Verification items for the finished model (mm, model axes). A direction names the side the tool comes from. Coordinates: 2 decimals unless noted, no trailing zeros. Write each loop counter-clockwise with the first axis right and the second up, starting at its lowest first coordinate (ties: lowest second). Pieces come first, ordered by that corner, then holes. Notation, with made-up numbers: (-16, 27) - (-1, 27) arc R30 ccw to (-1, 66) - close; hole circle Ø5 at (29, -1.5). An arc over 180 degrees is marked (long way). Use CSV: the item, a comma, the result in double quotes. Start each with the question number.
```python
from build123d import *

# Parameters (mm, degrees)
SKETCH1_W          = 6.5
SKETCH1_H          = 15
SKETCH2_R          = 4.5
CUT_EXTRUDE1_DEPTH = 13
SKETCH3_R          = 2
CUT_EXTRUDE2_DEPTH = 13


with BuildPart() as part:
    # Sketch1 → Revolve1 (revolve)
    with BuildSketch(Plane.XY, mode=Mode.PRIVATE) as revolve1_sk:
        with Locations((3.25, 0)):
            Rectangle(SKETCH1_W, SKETCH1_H)
    revolve(revolve1_sk.sketch.rotate(Axis((0, 7.5, 0), (0, -1, 0)), 90), axis=Axis((0, 7.5, 0), (0, -1, 0)))

    # Sketch2 → Cut-Extrude1 (cut)
    with BuildSketch(Plane.XZ.offset(7.5)):
        with Locations(Location((0, 0, 0), (0, 0, 270))):
            Circle(SKETCH2_R)
    extrude(amount=-CUT_EXTRUDE1_DEPTH, mode=Mode.SUBTRACT)

    # Sketch3 → Cut-Extrude2 (cut)
    with BuildSketch(Plane.XY):
        Circle(SKETCH3_R)
    extrude(amount=-CUT_EXTRUDE2_DEPTH, mode=Mode.SUBTRACT)


solid = part.part
```
Q1. Scan lines: line 1 along Y through (x, z) = (0, -5.1); line 2 along Y through (x, z) = (-2.75, -2); line 3 along Z through (x, y) = (3.75, -4.5). Record each from-to range of solid material in increasing order. Write a range as from..to.
Q2. Cross-section at D-D (x = 1.5). Record the cut outline in (y, z), plus the area to 3 significant figures.
Q3. Release check for a two-part mould opening along X. For faces 3 (the flat face through (-1.54, -7.5, 4.42)), 4 (the cylindrical face through (1.847, -0.766, -5.248)), 5 (the flat face through (0, 5.5, 0)), 6 (the cylindrical face through (-1.95, 0.11, 6.2)) record: released by +X, released by -X, zero draft, split by the parting line, or undercut.
Q4. Cross-section at B-B (z = 0). Record the cut outline in (x, y).
Q5. Cross-section at A-A (x = 0). Record the cut outline in (y, z), plus the area to 3 significant figures.
Q6. Gauge pin test, flat ends, axial feed: pin 1 (1.5 mm diameter, centred on y = -4, z = 5, fed in from -X); pin 2 (2 mm diameter, centred on x = -2, y = -2, fed in from -Z); pin 3 (2 mm diameter, centred on y = -6, z = -4.5, fed in from +X). Record the tip position at first contact, or that the pin passes through.
Q7. Cross-section at C-C (y = -6). Record the cut outline in (x, z).
Q8. Tool access check on faces 1 (the cylindrical face through (0.198, -1.091, 4.496)), 2 (the flat face through (0, 7.5, 0)). Record the directions out of +Z, -Z, +X, -X, +Y, -Y that give a thin tool (end or side, any length) a straight path to the whole face; none if there is none.
Reply:
1,line 1,"-7.5..-2, 2..7.5"
1,line 2,"5.5..7.5"
1,line 3,"-5.31..-2.49, 2.49..5.31"
2,outline,"(-7.5, -6.32) - (-1.32, -6.32) - (-1.32, -4.24) - (-7.5, -4.24) - close; (-7.5, 4.24) - (5.5, 4.24) - (5.5, -4.24) - (1.32, -4.24) - (1.32, -6.32) - (7.5, -6.32) - (7.5, 6.32) - (-7.5, 6.32) - close"
2,area,"73.9 mm^2"
3,face 3,"zero draft"
3,face 4,"undercut"
3,face 5,"undercut"
3,face 6,"split by the parting line"
4,outline,"(-6.5, -7.5) - (-4.5, -7.5) - (-4.5, 5.5) - (4.5, 5.5) - (4.5, -7.5) - (6.5, -7.5) - (6.5, 7.5) - (-6.5, 7.5) - close"
5,outline,"(-7.5, -6.5) - (-2, -6.5) - (-2, -4.5) - (-7.5, -4.5) - close; (-7.5, 4.5) - (5.5, 4.5) - (5.5, -4.5) - (2, -4.5) - (2, -6.5) - (7.5, -6.5) - (7.5, 6.5) - (-7.5, 6.5) - close"
5,area,"70.0 mm^2"
6,pin 1,"x = -4.92"
6,pin 2,"z = -6.42"
6,pin 3,"x = 5.48"
7,outline,"circle Ø13 at (0, 0); hole circle Ø9 at (0, 0)"
8,face 1,"-Y"
8,face 2,"+Z, -Z, +X, -X, +Y"
